Check sheet for the modelled part. Datum: model origin and axes. Units: mm. A direction names the side the tool comes from. Give positions to 0.01 mm unless a question says otherwise; leave off trailing zeros. Order: outer loops, then holes, each group sorted by start corner. A loop starts at its lowest first (then second) coordinate and runs counter-clockwise, first axis right, second up. Notation, with made-up numbers: (85, 23) - (123, 23) arc R33 cw to (123, 56) - close; hole circle Ø1 at (30, 48.25). An arc over 180 degrees is marked (long way). Answer in a Markdown table with one row per item.
from build123d import *

# Parameters (mm, degrees)
SKETCH2_R           = 5.588
BOSS_EXTRUDE1_DEPTH = 222.25
SKETCH3_R           = 3.937
BOSS_EXTRUDE2_DEPTH = 12.7
BOSS_EXTRUDE3_START = 12.7
SKETCH4_R           = 3.937
BOSS_EXTRUDE3_DEPTH = 12.7
SKETCH5_R           = 1.143
CUT_EXTRUDE1_DEPTH  = 25.4
CUT_EXTRUDE2_START  = -25.4
SKETCH6_R           = 1.143
CUT_EXTRUDE2_DEPTH  = 25.4
CHAMFER2_SIZE       = 0.762


with BuildPart() as part:
    # Sketch2 → Boss-Extrude1 (new, symmetric)
    with BuildSketch(Plane.XY):
        Circle(SKETCH2_R)
    extrude(amount=BOSS_EXTRUDE1_DEPTH, both=True)

    # Sketch3 → Boss-Extrude2 (add)
    with BuildSketch(Plane.XY.offset(222.25)):
        Circle(SKETCH3_R)
    extrude(amount=BOSS_EXTRUDE2_DEPTH)

    # Sketch4 → Boss-Extrude3 (add)
    with BuildSketch(Plane(origin=(0, 0, -222.25), x_dir=(-1, 0, 0), z_dir=(0, 0, -1)).offset(BOSS_EXTRUDE3_START)):
        with Locations(Location((0, 0, 0), (0, 0, 180))):
            Circle(SKETCH4_R)
    extrude(amount=-BOSS_EXTRUDE3_DEPTH)

    # Sketch5 → Cut-Extrude1 (cut)
    with BuildSketch(Plane.XY.offset(234.95)):
        Circle(SKETCH5_R)
    extrude(amount=-CUT_EXTRUDE1_DEPTH, mode=Mode.SUBTRACT)

    # Sketch6 → Cut-Extrude2 (cut)
    with BuildSketch(Plane(origin=(0, 0, -234.95), x_dir=(-1, 0, 0), z_dir=(0, 0, -1)).offset(CUT_EXTRUDE2_START)):
        with Locations(Location((0, 0, 0), (0, 0, 180))):
            Circle(SKETCH6_R)
    extrude(amount=CUT_EXTRUDE2_DEPTH, mode=Mode.SUBTRACT)

    # Chamfer2
    chamfer2_edges = [part.edges().sort_by_distance(p)[0] for p in [
        (-3.937, 0, -234.95),
        (-3.937, 0, 234.95),
    ]]
    chamfer(chamfer2_edges, length=CHAMFER2_SIZE)


solid = part.part
(1) Gauge pin test, flat ends, axial feed: P1, Ø2, axis at x = 3.5, z = -98.5, coming from the +Y side; P2, Ø0.7, axis at x = -0.5, y = -0.5, coming from the +Z side; P3, Ø4, axis at x = -4.5, y = 4, coming from the +Z side. Record the tip position at first contact, or that the pin passes through.
Geometry says:
| item | result |
|---|---|
| P1 | y = 5 |
| P2 | z = 209.55 |
| P3 | z = 222.25 |
(2) Thickness scan on L1, parallel to Y at x = 0, z = -225.25; L2, parallel to Y at x = 0, z = 218.75; L3, parallel to Y at x = -0.5, z = 181.5. Record the ranges inside material, lowest first.
Geometry says:
| item | result |
|---|---|
| L1 | -3.94 to -1.14, 1.14 to 3.94 |
| L2 | -5.59 to -1.14, 1.14 to 5.59 |
| L3 | -5.57 to 5.57 |
(3) Access from +Z, -Z, +X, -X, +Y, -Y to the whole of each face (thin tool, end or side, straight path). Record for faces 1 (the cylindrical face through (-0.853, -3.843, 228.135)), 2 (the cylindrical face through (-4.434, -3.4, 3.112)), 3 (the cylindrical face through (-0.853, 3.843, -228.303)).
Geometry says:
| item | result |
|---|---|
| face 1 | +Z |
| face 2 | +Z, -Z |
| face 3 | -Z |
(4) Cross-section at A-A, the plane z = 121.5. Record the cut outline in (x, y), then the cut area to 3 significant figures.
Geometry says:
| item | result |
|---|---|
| outline | circle Ø11.18 at (0, 0) |
| area | 98.1 mm² |
